Could you check a few things on this model? Use its own coordinates, in mm. Coordinates: 2 decimals unless noted, no trailing zeros. Order: outer loops, then holes, each group sorted by start corner. A loop starts at its lowest first (then second) coordinate and runs counter-clockwise, first axis right, second up. Notation, with made-up numbers: (-40, 25.5) -> (-31, 25.5) arc R13 cw to (-31, 49.5) -> close; hole circle Ø11 at (-10, 26). An arc over 180 degrees is marked (long way). Use a Markdown table: item, result. Add a question column.
1) Will these pins go through, and if not, where does the flat tip stop? pin 1 Ø5.5 at (x, y) = (72, -62) entering from +Z; pin 2 Ø4 at (x, y) = (-470, 56) entering from -Z; pin 3 Ø8 at (y, z) = (67.5, 4.5) entering from -X; pin 4 Ø6 at (x, z) = (-508.5, 6) entering from -Y.
2) If we section it at B-B (x = -532): Write out the boundary of the cut face in (y, z).
3) If I drill on L1, parallel to Y at x = -170, z = -0.5; L2, parallel to Y at x = -225, z = -3; L3, parallel to Y at x = -690, z = -2.25, over which ranges is the centre line in solid material (lowest first)? Write a range as [from, to].
4) If we section it at A-A (z = 0.25): Give the number of separate pieces and of enclosed holes in the cut face, plus the area to 3 significant figures.
```python
from build123d import *

# Parameters (mm, degrees)
SKIZZE1_R                                            = 2.5
AUFSATZ_LINEAR_AUSTRAGEN1_DEPTH                      = 7.5
M6_GEWINDEBOHRUNG1_D                                 = 5
M8_GEWINDEBOHRUNG1_D                                 = 6.8
DURCHGANGSLOCH_F_R_M81_D                             = 9
F_5_0_5_DURCHMESSER_BOHRUNG1_D                       = 5
STIRNSENKUNG_F_R_M6_ZYLINDERSCHRAUBE_MIT_D           = 6.6
STIRNSENKUNG_F_R_M6_ZYLINDERSCHRAUBE_MIT_CBORE_D     = 11
STIRNSENKUNG_F_R_M6_ZYLINDERSCHRAUBE_MIT_CBORE_DEPTH = 4.4
F_7_0_7_DURCHMESSER_BOHRUNG2_D                       = 7
M6_GEWINDEBOHRUNG2_D                                 = 5


with BuildPart() as part:
    # Skizze1 → Aufsatz-Linear austragen1 (new, symmetric)
    with BuildSketch(Plane.XY):
        with BuildLine():
            Line((0, 40), (75, 40))
            ThreePointArc((75, 40), (78.535533906, 41.464466094), (80, 45))
            Line((80, 45), (80, 86))
            ThreePointArc((80, 86), (78.535533906, 89.535533906), (75, 91))
            Line((75, 91), (-605.785553141, 91))
            ThreePointArc((-605.785553141, 91), (-608.373743593, 90.659258263), (-610.785553141, 89.660254038))
            Line((-610.785553141, 89.660254038), (-694, 41.616370744))
            ThreePointArc((-694, 41.616370744), (-698.392304845, 37.224065898), (-700, 31.224065898))
            Line((-700, 31.224065898), (-700, -3.445240413))
            ThreePointArc((-700, -3.445240413), (-697.829824531, -10.328157649), (-692.10424172, -14.721551862))
            Line((-692.10424172, -14.721551862), (-503.420201433, -83.396926208))
            ThreePointArc((-503.420201433, -83.396926208), (-501.736481777, -83.84807753), (-500, -84))
            Line((-500, -84), (-61.111641217, -84))
            ThreePointArc((-61.111641217, -84), (-60.057548663, -83.8876261), (-59.050837107, -83.555555556))
            ThreePointArc((-59.050837107, -83.555555556), (-50.997144653, -80.898991204), (-42.564404226, -80))
            Line((-42.564404226, -80), (6.561649764, -80))
            ThreePointArc((6.561649764, -80), (6.997428478, -79.98097349), (7.429890653, -79.924038765))
            Line((7.429890653, -79.924038765), (75.868240888, -67.856511103))
            ThreePointArc((75.868240888, -67.856511103), (78.830222216, -66.146410387), (80, -62.932472338))
            Line((80, -62.932472338), (80, -45))
            ThreePointArc((80, -45), (78.535533906, -41.464466094), (75, -40))
            Line((75, -40), (0, -40))
            ThreePointArc((0, -40), (-40, 0), (0, 40))
        make_face()
        with Locations((-690, 30)):
            Circle(SKIZZE1_R, mode=Mode.SUBTRACT)
        with Locations((-590, -2)):
            Circle(SKIZZE1_R, mode=Mode.SUBTRACT)
    extrude(amount=AUFSATZ_LINEAR_AUSTRAGEN1_DEPTH, both=True)

    # M6 Gewindebohrung1 (through all)
    with Locations(Plane.XY.offset(7.5)):
        with Locations((-590, 30), (-690, -2), (-642, 61), (-642, -19)):
            Hole(M6_GEWINDEBOHRUNG1_D / 2)

    # M8 Gewindebohrung1 (through all)
    with Locations(Plane.XY.offset(7.5)):
        with Locations((-24.874423104, -60.052169613), (-24.874423104, 60.052169613), (24.874423104, 60.052169613), (24.874423104, -60.052169613)):
            Hole(M8_GEWINDEBOHRUNG1_D / 2)

    # Durchgangsloch für M81 (through all)
    with Locations(Plane.XY.offset(7.5)):
        with Locations((-500, -64), (-110, -64)):
            Hole(DURCHGANGSLOCH_F_R_M81_D / 2)

    # Ø5.0 (5) Durchmesser Bohrung1 (through all)
    with Locations(Plane.XY.offset(7.5)):
        with Locations((-170, 27), (-470, 27)):
            Hole(F_5_0_5_DURCHMESSER_BOHRUNG1_D / 2)

    # Stirnsenkung für M6 Zylinderschraube mit Innensechskant1 (through all)
    with Locations(Plane.XY.offset(7.5)):
        with Locations((70, 60), (70, -60)):
            stirnsenkung_f_r_m6_zylinderschraube_mit = CounterBoreHole(STIRNSENKUNG_F_R_M6_ZYLINDERSCHRAUBE_MIT_D / 2, STIRNSENKUNG_F_R_M6_ZYLINDERSCHRAUBE_MIT_CBORE_D / 2, STIRNSENKUNG_F_R_M6_ZYLINDERSCHRAUBE_MIT_CBORE_DEPTH)

    # Spiegeln1: Stirnsenkung für M6 Zylinderschraube mit Innensechskant1 across plane
    add(stirnsenkung_f_r_m6_zylinderschraube_mit.mirror(Plane.XY), mode=Mode.SUBTRACT)

    # Ø7.0 (7) Durchmesser Bohrung2 (through all)
    with Locations(Plane.XY.offset(7.5)):
        with Locations((-75, 56), (-225, 56), (-340, 56), (-470, 56), (-600, 56)):
            Hole(F_7_0_7_DURCHMESSER_BOHRUNG2_D / 2)

    # M6 Gewindebohrung2 (through all)
    with Locations(Plane(origin=(0, 0, -7.5), x_dir=(-1, 0, 0), z_dir=(0, 0, -1))):
        with Locations((81, -75), (401, -75)):
            Hole(M6_GEWINDEBOHRUNG2_D / 2)


solid = part.part
```
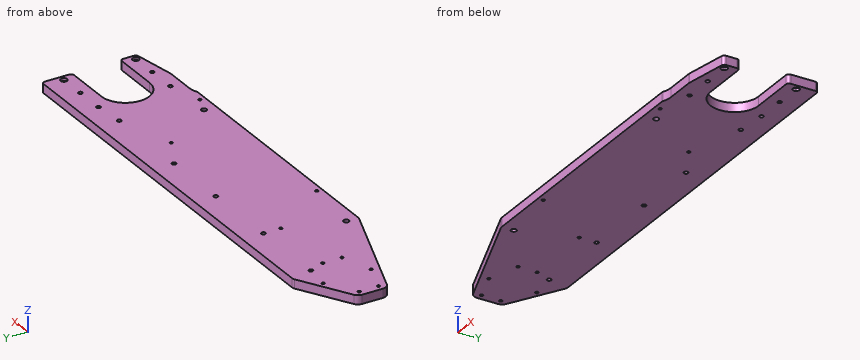
Answer sheet:
| question | item | result |
|---|---|---|
| 1 | pin 1 | z = 7.5 |
| 1 | pin 2 | through |
| 1 | pin 3 | x = -656.1 |
| 1 | pin 4 | y = -82.64 |
| 2 | outline | (-72.99, -7.5) -> (91, -7.5) -> (91, 7.5) -> (-72.99, 7.5) -> close |
| 3 | L1 | [-84, 24.5], [29.5, 91] |
| 3 | L2 | [-84, 52.5], [59.5, 91] |
| 3 | L3 | [-15.49, -4.5], [0.5, 27.5], [32.5, 43.93] |
| 4 | separate pieces | 1 |
| 4 | enclosed holes | 23 |
| 4 | area | 116,000 mm2 |
